```python
from build123d import *

# Parameters (mm, degrees)
CUT_EXTRUDE_1_REACH      = 256.755
SKETCH_2_R               = 2.5
PATTERN_CIRCULAR_1_COUNT = 12
SKETCH_3_W               = 60
SKETCH_3_H               = 45
EXTRUDE_1_DEPTH          = 8
CUT_EXTRUDE_2_REACH      = 330.786
SKETCH_4_R               = 10
SKETCH_4_R_2             = 1.3
CUT_EXTRUDE_3_REACH      = 330.786
SKETCH_5_R               = 1.3
SKETCH_5_W               = 12
SKETCH_5_H               = 22


with BuildPart() as part:
    # Sketch 1 → Revolve 1 (revolve)
    with BuildSketch(Plane(origin=(0, 0, 0), x_dir=(0, 0, -1), z_dir=(1, 0, 0)), mode=Mode.PRIVATE) as revolve_1_sk:
        Polygon((0, 0), (108, 0), (108, 10), (120, 10), (120, 190), (116, 190), (116, 180), (96, 180), (96, 175), (116, 175), (116, 15), (104, 15), (104, 5), (0, 5), align=None)
    revolve(revolve_1_sk.sketch.rotate(Axis((0, 5, 0), (0, -1, 0)), 180), axis=Axis((0, 5, 0), (0, -1, 0)))

    # Sketch 2 → Cut-Extrude 1 (cut, up to next)
    with BuildSketch(Plane.XZ, mode=Mode.PRIVATE) as cut_extrude_1_sk1:
        with Locations(Location((0, -15, 0), (0, 0, 270))):
            Circle(SKETCH_2_R)
    cut_extrude_1_tool1 = extrude(cut_extrude_1_sk1.sketch, amount=-CUT_EXTRUDE_1_REACH, mode=Mode.PRIVATE) & part.part
    # Sketch 2 → Cut-Extrude 1 (cut, up to next)
    with BuildSketch(Plane.XZ, mode=Mode.PRIVATE) as cut_extrude_1_sk2:
        with Locations(Location((0, -25, 0), (0, 0, 270))):
            Circle(SKETCH_2_R)
    cut_extrude_1_tool2 = extrude(cut_extrude_1_sk2.sketch, amount=-CUT_EXTRUDE_1_REACH, mode=Mode.PRIVATE) & part.part
    # Sketch 2 → Cut-Extrude 1 (cut, up to next)
    with BuildSketch(Plane.XZ, mode=Mode.PRIVATE) as cut_extrude_1_sk3:
        with Locations(Location((0, -35, 0), (0, 0, 270))):
            Circle(SKETCH_2_R)
    cut_extrude_1_tool3 = extrude(cut_extrude_1_sk3.sketch, amount=-CUT_EXTRUDE_1_REACH, mode=Mode.PRIVATE) & part.part
    # Sketch 2 → Cut-Extrude 1 (cut, up to next)
    with BuildSketch(Plane.XZ, mode=Mode.PRIVATE) as cut_extrude_1_sk4:
        with Locations(Location((0, -45, 0), (0, 0, 270))):
            Circle(SKETCH_2_R)
    cut_extrude_1_tool4 = extrude(cut_extrude_1_sk4.sketch, amount=-CUT_EXTRUDE_1_REACH, mode=Mode.PRIVATE) & part.part
    # Sketch 2 → Cut-Extrude 1 (cut, up to next)
    with BuildSketch(Plane.XZ, mode=Mode.PRIVATE) as cut_extrude_1_sk5:
        with Locations(Location((0, -55, 0), (0, 0, 270))):
            Circle(SKETCH_2_R)
    cut_extrude_1_tool5 = extrude(cut_extrude_1_sk5.sketch, amount=-CUT_EXTRUDE_1_REACH, mode=Mode.PRIVATE) & part.part
    # Sketch 2 → Cut-Extrude 1 (cut, up to next)
    with BuildSketch(Plane.XZ, mode=Mode.PRIVATE) as cut_extrude_1_sk6:
        with Locations(Location((0, -65, 0), (0, 0, 270))):
            Circle(SKETCH_2_R)
    cut_extrude_1_tool6 = extrude(cut_extrude_1_sk6.sketch, amount=-CUT_EXTRUDE_1_REACH, mode=Mode.PRIVATE) & part.part
    # Sketch 2 → Cut-Extrude 1 (cut, up to next)
    with BuildSketch(Plane.XZ, mode=Mode.PRIVATE) as cut_extrude_1_sk7:
        with Locations(Location((0, -75, 0), (0, 0, 270))):
            Circle(SKETCH_2_R)
    cut_extrude_1_tool7 = extrude(cut_extrude_1_sk7.sketch, amount=-CUT_EXTRUDE_1_REACH, mode=Mode.PRIVATE) & part.part
    cut_extrude_1_1 = cut_extrude_1_tool1.solids().sort_by_distance((0, 0, -15))[0]
    add(cut_extrude_1_1, mode=Mode.SUBTRACT)
    cut_extrude_1_2 = cut_extrude_1_tool2.solids().sort_by_distance((0, 0, -25))[0]
    add(cut_extrude_1_2, mode=Mode.SUBTRACT)
    cut_extrude_1_3 = cut_extrude_1_tool3.solids().sort_by_distance((0, 0, -35))[0]
    add(cut_extrude_1_3, mode=Mode.SUBTRACT)
    cut_extrude_1_4 = cut_extrude_1_tool4.solids().sort_by_distance((0, 0, -45))[0]
    add(cut_extrude_1_4, mode=Mode.SUBTRACT)
    cut_extrude_1_5 = cut_extrude_1_tool5.solids().sort_by_distance((0, 0, -55))[0]
    add(cut_extrude_1_5, mode=Mode.SUBTRACT)
    cut_extrude_1_6 = cut_extrude_1_tool6.solids().sort_by_distance((0, 0, -65))[0]
    add(cut_extrude_1_6, mode=Mode.SUBTRACT)
    cut_extrude_1_7 = cut_extrude_1_tool7.solids().sort_by_distance((0, 0, -75))[0]
    add(cut_extrude_1_7, mode=Mode.SUBTRACT)
    cut_extrude_1 = cut_extrude_1_1 + cut_extrude_1_2 + cut_extrude_1_3 + cut_extrude_1_4 + cut_extrude_1_5 + cut_extrude_1_6 + cut_extrude_1_7  # Cut-Extrude 1 as one shape, for the pattern or mirror that repeats it

    # Pattern Circular 1: Cut-Extrude 1 ×12 about axis
    pattern_circular_1_axis = Axis((0, 0, 0), (0, 1, 0))
    for i in range(1, PATTERN_CIRCULAR_1_COUNT):
        add(cut_extrude_1.rotate(pattern_circular_1_axis, i * 360 / PATTERN_CIRCULAR_1_COUNT), mode=Mode.SUBTRACT)

    # Sketch 3 → Extrude 1 (add)
    with BuildSketch(Plane(origin=(0, 0, -120), x_dir=(-1, 0, 0), z_dir=(0, 0, -1))):
        with Locations((0, 67.5)):
            Rectangle(SKETCH_3_W, SKETCH_3_H)
    extrude(amount=-EXTRUDE_1_DEPTH)

    # Sketch 4 → Cut-Extrude 2 (cut, up to next)
    with BuildSketch(Plane(origin=(0, 0, -120), x_dir=(-1, 0, 0), z_dir=(0, 0, -1)), mode=Mode.PRIVATE) as cut_extrude_2_sk1:
        with Locations((15, 75)):
            Circle(SKETCH_4_R)
    cut_extrude_2_tool1 = extrude(cut_extrude_2_sk1.sketch, amount=-CUT_EXTRUDE_2_REACH, mode=Mode.PRIVATE) & part.part
    # Sketch 4 → Cut-Extrude 2 (cut, up to next)
    with BuildSketch(Plane(origin=(0, 0, -120), x_dir=(-1, 0, 0), z_dir=(0, 0, -1)), mode=Mode.PRIVATE) as cut_extrude_2_sk2:
        with Locations((24.75, 81.7)):
            Circle(SKETCH_4_R_2)
    cut_extrude_2_tool2 = extrude(cut_extrude_2_sk2.sketch, amount=-CUT_EXTRUDE_2_REACH, mode=Mode.PRIVATE) & part.part
    # Sketch 4 → Cut-Extrude 2 (cut, up to next)
    with BuildSketch(Plane(origin=(0, 0, -120), x_dir=(-1, 0, 0), z_dir=(0, 0, -1)), mode=Mode.PRIVATE) as cut_extrude_2_sk3:
        with Locations((5.25, 81.7)):
            Circle(SKETCH_4_R_2)
    cut_extrude_2_tool3 = extrude(cut_extrude_2_sk3.sketch, amount=-CUT_EXTRUDE_2_REACH, mode=Mode.PRIVATE) & part.part
    # Sketch 4 → Cut-Extrude 2 (cut, up to next)
    with BuildSketch(Plane(origin=(0, 0, -120), x_dir=(-1, 0, 0), z_dir=(0, 0, -1)), mode=Mode.PRIVATE) as cut_extrude_2_sk4:
        with Locations((5.25, 47.7)):
            Circle(SKETCH_4_R_2)
    cut_extrude_2_tool4 = extrude(cut_extrude_2_sk4.sketch, amount=-CUT_EXTRUDE_2_REACH, mode=Mode.PRIVATE) & part.part
    # Sketch 4 → Cut-Extrude 2 (cut, up to next)
    with BuildSketch(Plane(origin=(0, 0, -120), x_dir=(-1, 0, 0), z_dir=(0, 0, -1)), mode=Mode.PRIVATE) as cut_extrude_2_sk5:
        with Locations((24.75, 47.7)):
            Circle(SKETCH_4_R_2)
    cut_extrude_2_tool5 = extrude(cut_extrude_2_sk5.sketch, amount=-CUT_EXTRUDE_2_REACH, mode=Mode.PRIVATE) & part.part
    add(cut_extrude_2_tool1.solids().sort_by_distance((-15, 75, -120))[0], mode=Mode.SUBTRACT)
    add(cut_extrude_2_tool2.solids().sort_by_distance((-24.75, 81.7, -120))[0], mode=Mode.SUBTRACT)
    add(cut_extrude_2_tool3.solids().sort_by_distance((-5.25, 81.7, -120))[0], mode=Mode.SUBTRACT)
    add(cut_extrude_2_tool4.solids().sort_by_distance((-5.25, 47.7, -120))[0], mode=Mode.SUBTRACT)
    add(cut_extrude_2_tool5.solids().sort_by_distance((-24.75, 47.7, -120))[0], mode=Mode.SUBTRACT)

    # Sketch 5 → Cut-Extrude 3 (cut, up to next)
    with BuildSketch(Plane(origin=(0, 0, -120), x_dir=(-1, 0, 0), z_dir=(0, 0, -1)), mode=Mode.PRIVATE) as cut_extrude_3_sk1:
        with Locations((-19, 87)):
            Circle(SKETCH_5_R)
    cut_extrude_3_tool1 = extrude(cut_extrude_3_sk1.sketch, amount=-CUT_EXTRUDE_3_REACH, mode=Mode.PRIVATE) & part.part
    # Sketch 5 → Cut-Extrude 3 (cut, up to next)
    with BuildSketch(Plane(origin=(0, 0, -120), x_dir=(-1, 0, 0), z_dir=(0, 0, -1)), mode=Mode.PRIVATE) as cut_extrude_3_sk2:
        with Locations((-19, 60.5)):
            Circle(SKETCH_5_R)
    cut_extrude_3_tool2 = extrude(cut_extrude_3_sk2.sketch, amount=-CUT_EXTRUDE_3_REACH, mode=Mode.PRIVATE) & part.part
    # Sketch 5 → Cut-Extrude 3 (cut, up to next)
    with BuildSketch(Plane(origin=(0, 0, -120), x_dir=(-1, 0, 0), z_dir=(0, 0, -1)), mode=Mode.PRIVATE) as cut_extrude_3_sk3:
        with Locations((-19, 74)):
            Rectangle(SKETCH_5_W, SKETCH_5_H)
    cut_extrude_3_tool3 = extrude(cut_extrude_3_sk3.sketch, amount=-CUT_EXTRUDE_3_REACH, mode=Mode.PRIVATE) & part.part
    add(cut_extrude_3_tool1.solids().sort_by_distance((19, 87, -120))[0], mode=Mode.SUBTRACT)
    add(cut_extrude_3_tool2.solids().sort_by_distance((19, 60.5, -120))[0], mode=Mode.SUBTRACT)
    add(cut_extrude_3_tool3.solids().sort_by_distance((19, 74, -120))[0], mode=Mode.SUBTRACT)


solid = part.part
```
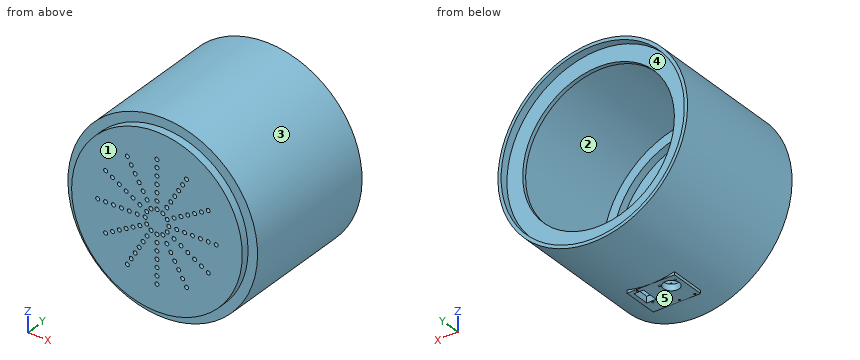
The model under review builds one solid part; all positions refer to its coordinate system, in mm. Face numbers are marked on the shaded views. A direction names the side the tool comes from. Round coordinates to 2 decimals unless told otherwise and drop trailing zeros. Order: outer loops, then holes, each group sorted by start corner. A loop starts at its lowest first (then second) coordinate and runs counter-clockwise, first axis right, second up.
Item 1: For pin 1 (3 mm diameter, centred on x = 0, z = -15, fed in from +Y); pin 2 (4 mm diameter, centred on x = -43, y = 91, fed in from +Z); pin 3 (4 mm diameter, centred on x = 46, y = 22, fed in from +Z); pin 4 (1 mm diameter, centred on x = -16.5, y = 170.5, fed in from +Z), all flat-tipped, find the tip position at first contact; note any pin that passes through.
Working result:
pin 1: passes through
pin 2: stops at z = 112.78
pin 3: stops at z = 111.64
pin 4: stops at z = 118.93
Item 2: Draft analysis for pull direction X (two halves, no side actions). For the marked faces 1, 2 and 3, state which applies: released by +X, released by -X, zero draft, split by the parting line, or undercut.
Working result:
face 1: zero draft
face 2: undercut
face 3: split by the parting line
Item 3: Machinability: for the marked faces 4 and 5, which of the approach directions +Z, -Z, +X, -X, +Y, -Y give a long, thin tool a straight path to every point of the face, cutting with its end or side? Answer none if there is none.
Working result:
face 4: +Y
face 5: -Z, +X, -X, +Y, -Y
Item 4: Add section B-B, the plane x = -86. State the section outline as (y, z) points, and give its area (3 significant figures).
Working result:
outline: (0, -65.33) - (10, -65.33) - (10, -83.69) - (190, -83.69) - (190, -77.85) - (180, -77.85) - (180, -42.66) - (175, -42.66) - (175, -77.85) - (15, -77.85) - (15, -58.48) - (5, -58.48) - (5, 58.48) - (15, 58.48) - (15, 77.85) - (175, 77.85) - (175, 42.66) - (180, 42.66) - (180, 77.85) - (190, 77.85) - (190, 83.69) - (10, 83.69) - (10, 65.33) - (0, 65.33) - close
area: 3,370 mm2
Item 5: Add section A-A, the plane y = 68.5. State the section outline as (x, z) points.
Working result:
outline: (-30, -120) - (-22.6, -120) - (-22.6, -112) - (-30, -112) - (-30, -112.05) arc R116 cw (long way) to (30, -112.05) - (30, -112) - (25, -112) - (25, -120) - (30, -120) - (30, -116.19) arc R120 ccw (long way) to (-30, -116.19) - close; (-7.4, -120) - (13, -120) - (13, -112) - (-7.4, -112) - close
Item 6: To check wall thickness, follow probe 1 along Z at (x, y) = (-55, 1.1); probe 2 along X at (y, z) = (3, -7.5); probe 3 along Y at (x, z) = (15, -46). State the ranges of each line that lie inside material, in increasing order.
Working result:
probe 1: z = -92.95 to -34.64, -30.36 to -2.5, 2.5 to 30.36, 34.64 to 92.95
probe 2: x = -107.74 to -15.49, -10.49 to 10.49, 15.49 to 107.74
probe 3: y = 0 to 5
